Read the model definition and answer for the solid it produces. Units are mm, in the model's axes. Face numbers are marked on the shaded views. A direction names the side the tool comes from. Coordinates: 2 decimals unless noted, no trailing zeros. Loops run counter-clockwise (first coordinate to the right, second up) from the corner with the lowest first, then second, coordinate; pieces in that order, holes last. Notation, with made-up numbers: M 41,58.5 L 71,58.5 A20 ccw 71,89.5 Z; hole C -28,25 d10. An arc over 180 degrees is marked long. One line per item, written item: value. Start each with the question number.
1. Flat-ended cylindrical pins translate along their axes: pin 1 (1.5 mm diameter, centred on y = 17.5, z = 6, fed in from +X); pin 2 (1 mm diameter, centred on x = -17.5, y = 12.5, fed in from +Z) (1 decimal); pin 3 (8 mm diameter, centred on x = 15, y = 37, fed in from +Z); pin 4 (11 mm diameter, centred on x = -15, y = 37, fed in from +Z). Find the tip coordinate at first contact, or state that the pin passes through.
2. For the marked faces 4, 5 and 6, determine the directions among +Z, -Z, +X, -X, +Y, -Y from which every point of the face is accessible in a straight line to the end or side of a thin tool.
3. The part is cut by section B-B (z = 0). Write down the section's boundary in (x, y).
4. The part is cut by section D-D (x = 15). Write down the section's boundary in (y, z), then the cut area to 3 significant figures.
5. Determine the mould class of the marked faces 1, 2 and 3 for opening direction X: +X half, -X half, draft (parallel to the pull), parting line (faces both ways), or undercut.
6. The part is cut by section A-A (x = 0). Write down the section's boundary in (y, z), then the cut area to 4 significant figures.
7. The part is cut by section C-C (y = 12). Write down the section's boundary in (x, z).
8. Consider probe 1 along Y at (x, z) = (15, 2.5); probe 2 along X at (y, z) = (37, -3.5); probe 3 along X at (y, z) = (12, -3.25). Determine where each line is inside the solid, lowest interval first.
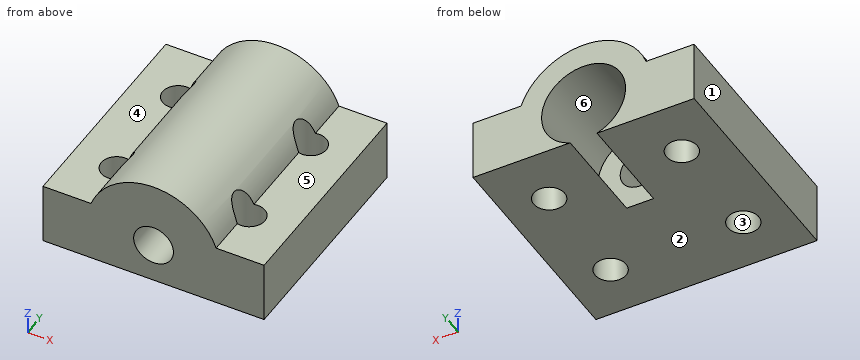
Autodesk Fusion 360 part; units mm, degrees
sketch "Sketch1" plane through (0, 0, 0) normal (0, 1, 0) x (1, 0, 0)
  circle A0 centre (0, 0) radius 15
  circle A1 centre (0, 0) radius 4.5
  line L0 (-12, 9) -> (12, 9)
  line L1 (-12, 9) -> (-25, 9)
  line L2 (-25, 9) -> (-25, -5)
  line L3 (-25, -5) -> (25, -5)
  line L4 (25, -5) -> (25, 9)
  line L5 (25, 9) -> (12, 9)
  dimension "d1" = 9
  dimension "d2" = 30
  dimension "d3" = 9
  dimension "d6" = 25
  dimension "d7" = 25
  dimension "d8" = 14
extrude "Extrude1" add sketch "Sketch1" along normal blind 50 contours A0 L0 L3 | A0 L3 L4 L5 | A0 L3 | A0 L1 L2 L3
sketch "Sketch2" plane through (0, 0, -9) normal (0, 0, -1) x (1, 0, 0)
  line L0 (25, 0) -> (-25, 0)
  line L1 (-25, 0) -> (-25, -50)
  line L2 (-25, -50) -> (25, -50)
  line L3 (25, -50) -> (25, 0)
  line L4 (0, 0) -> (0, -50)
  circle A0 centre (-15, -12) radius 3.5
  circle A1 centre (-15, -37) radius 3.5
  circle A2 centre (15, -12) radius 3.5
  circle A3 centre (15, -37) radius 3.5
  dimension "d9" = 15
  dimension "d10" = 15
  dimension "d11" = 25
  dimension "d12" = 12
  dimension "d13" = 7
  dimension "d14" = 7
sketch "Sketch3" plane through (0, 50, 0) normal (0, 1, 0) x (-1, 0, 0)
  circle A0 centre (0, 0) radius 4.5
  line L0 (-25, -9) -> (25, -9)
  line L1 (25, -9) -> (25, 5)
  line L2 (25, 5) -> (14.1421, 5)
  arc A1 (14.1421, 5) -> (-14.1421, 5) centre (0, 0) ccw
  line L3 (-14.1421, 5) -> (-25, 5)
  line L4 (-25, 5) -> (-25, -9)
  circle A2 centre (0, 0) radius 9.5
  dimension "d15" = 19
sketch "Sketch4" plane through (0, 0, 5) normal (0, 0, 1) x (-1, 0, 0)
  line L0 (-14.1421, -50) -> (-14.1421, 0)
  line L1 (-14.1421, 0) -> (-25, 0)
  line L2 (-25, 0) -> (-25, -50)
  line L3 (-25, -50) -> (-14.1421, -50)
  line L4 (0, 0) -> (0, -41)
  line L5 (-14.1421, -15) -> (-25, -15)
  line L6 (-25, -15) -> (-25, 0)
  line L7 (-25, 0) -> (-14.1421, 0)
  line L8 (-14.1421, 0) -> (-14.1421, -15)
  line L9 (14.1421, -15) -> (25, -15)
  line L10 (14.1421, 0) -> (14.1421, -15)
  line L11 (25, 0) -> (14.1421, 0)
  line L12 (25, -15) -> (25, 0)
  dimension "d20" = 15
extrude "Extrude3" cut sketch "Sketch2" against normal blind 26 contours A0 | A1 | A2 | A3
extrude "Extrude2" cut sketch "Sketch3" against normal blind 23 contours L0 A2 picked at (-0.1121, -7.4958)
extrude "Extrude4" [suppressed]
equation "d7 = d6"
equation "d10 = d9"
equation "d14 = d13"
Answer block:
1. pin 1: stops at x = 14.05
1. pin 2: passes through
1. pin 3: stops at z = 10.2
1. pin 4: stops at z = 11.61
2. face 4: +Z, -X, +Y, -Y
2. face 5: +Z, +X, +Y, -Y
2. face 6: +Y
3. outline: M -25,0 L -4.5,0 L -4.5,27 L -9.5,27 L -9.5,50 L -25,50 Z; M 4.5,0 L 25,0 L 25,50 L 9.5,50 L 9.5,27 L 4.5,27 Z; hole C -15,12 d7; hole C -15,37 d7; hole C 15,12 d7; hole C 15,37 d7
4. outline: M 0,-9 L 8.5,-9 L 8.5,5 L 0,5 Z; M 15.5,-9 L 33.5,-9 L 33.5,5 L 15.5,5 Z; M 40.5,-9 L 50,-9 L 50,5 L 40.5,5 Z
4. area: 504 mm2
5. face 1: -X half
5. face 2: draft
5. face 3: undercut
6. outline: M 0,-9 L 27,-9 L 27,-4.5 L 0,-4.5 Z; M 0,4.5 L 27,4.5 L 27,9.5 L 50,9.5 L 50,15 L 0,15 Z
6. area: 531.5 mm2
7. outline: M -25,-9 L -18.5,-9 L -18.5,5 L -25,5 Z; M -11.5,-9 L 11.5,-9 L 11.5,9.63 A15 ccw -11.5,9.63 Z; M 18.5,-9 L 25,-9 L 25,5 L 18.5,5 Z; hole C 0,0 d9
8. probe 1: y = 0 to 8.5, 15.5 to 33.5, 40.5 to 50
8. probe 2: x = -25 to -18.5, -11.5 to -8.83, 8.83 to 11.5, 18.5 to 25
8. probe 3: x = -25 to -18.5, -11.5 to -3.11, 3.11 to 11.5, 18.5 to 25
